from build123d import *

# Parameters (mm, degrees)
SKETCH1_R           = 4
BOSS_EXTRUDE1_DEPTH = 15
CUT_EXTRUDE1_REACH  = 83.718
FILLET1_R           = 5


with BuildPart() as part:
    # Sketch1 → Boss-Extrude1 (new, symmetric)
    with BuildSketch(Plane.XY):
        with BuildLine():
            Line((-32.411165235, -2.9), (32.411165235, -2.9))
            ThreePointArc((32.411165235, -2.9), (36.084926186, -3.630756488), (39.199390335, -5.711774901))
            Line((39.199390335, -5.711774901), (51.448127676, -17.960512242))
            ThreePointArc((51.448127676, -17.960512242), (54.259902577, -24.748737342), (51.448127676, -31.536962441))
            Line((51.448127676, -31.536962441), (44.756401435, -38.228688682))
            ThreePointArc((44.756401435, -38.228688682), (38.472718241, -48.613591207), (48.857620766, -42.329908013))
            Line((48.857620766, -42.329908013), (55.549347007, -35.638181772))
            ThreePointArc((55.549347007, -35.638181772), (60.059902577, -24.748737342), (55.549347007, -13.859292911))
            Line((55.549347007, -13.859292911), (43.300609665, -1.61055557))
            ThreePointArc((43.300609665, -1.61055557), (38.304490094, 1.727744801), (32.411165235, 2.9))
            Line((32.411165235, 2.9), (-32.411165235, 2.9))
            Line((-32.411165235, 2.9), (-32.411165235, -2.9))
        make_face()
        with Locations((42.892135624, -44.194173824)):
            Circle(SKETCH1_R, mode=Mode.SUBTRACT)
    extrude(amount=BOSS_EXTRUDE1_DEPTH, both=True)

    # Sketch2 → Cut-Extrude1 (cut, up to next)
    with BuildSketch(Plane(origin=(0, 2.9, 0), x_dir=(1, 0, 0), z_dir=(0, 1, 0)), mode=Mode.PRIVATE) as cut_extrude1_sk1:
        with BuildLine():
            Line((-2.411165235, 3.5), (6.588834765, 3.5))
            ThreePointArc((6.588834765, 3.5), (10.088834765, 0), (6.588834765, -3.5))
            Line((6.588834765, -3.5), (-2.411165235, -3.5))
            ThreePointArc((-2.411165235, -3.5), (-5.911165235, 0), (-2.411165235, 3.5))
        make_face()
    cut_extrude1_tool1 = extrude(cut_extrude1_sk1.sketch, amount=-CUT_EXTRUDE1_REACH, mode=Mode.PRIVATE) & part.part
    add(cut_extrude1_tool1.solids().sort_by_distance((2.088835, 2.9, 0))[0], mode=Mode.SUBTRACT)

    # Fillet1
    fillet1_edges = [part.edges().sort_by_distance(p)[0] for p in [
        (-32.411165235, 0, -15),
        (-32.411165235, 0, 15),
    ]]
    fillet(fillet1_edges, radius=FILLET1_R)


solid = part.part
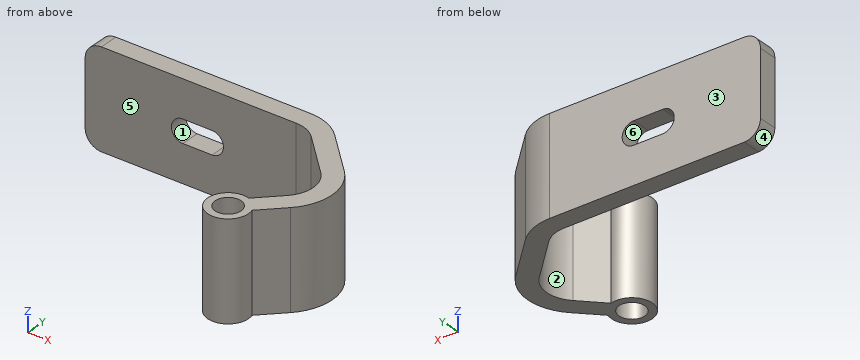
Here's how the part is built. I have some questions about the finished solid (model axes, mm). Face numbers are marked on the shaded views. A direction names the side the tool comes from. Round coordinates to 2 decimals unless told otherwise and drop trailing zeros. Order: outer loops, then holes, each group sorted by start corner. A loop starts at its lowest first (then second) coordinate and runs counter-clockwise, first axis right, second up. Notation, with made-up numbers: M 22,9.5 L 46,9.5 A25 ccw 46,38.5 Z; hole C 28,-24.5 d8. An arc over 180 degrees is marked long. Return JSON: item names as keys, results as strings. Group by question number.
1. I'm going to push flat-ended pins straight in: pin 1 Ø2 at (y, z) = (-7, 9) entering from -X; pin 2 Ø9 at (x, z) = (-8, 0.5) entering from -Y; pin 3 Ø6 at (y, z) = (-29.5, -7) entering from -X; pin 4 Ø7 at (x, y) = (42.89, -44.19) entering from +Z. Where does each tip first touch, or does it pass through?
2. If we mould it in two halves opening along Y, with no side actions, what happens to the marked faces 1, 2 and 3? For each: pulls with the +Y half, pulls with the -Y half, needs draft (parallel to the pull), parting line crosses it, or undercut.
3. If we section it at B-B on x = 2: List the corners of the cut face in (y, z) for me.
4. On a 3-axis mill with a long thin cutter (end or side, diameter ignored), from which of +Z, -Z, +X, -X, +Y, -Y can I reach the whole of each face in a straight line? I mean the marked faces 4, 5 and 6. Say none if no direction works.
5. If we section it at A-A on z = 0: List the corners of the cut face in (x, y) for me, then the cut area to 3 significant figures.
6. Please list where these lines run through material, in increasing order: probe 1 along Y at (x, z) = (-14.5, -11.5); probe 2 along Y at (x, z) = (46.5, 10.25); probe 3 along Y at (x, z) = (52, -10.5).
7. If we section it at C-C on z = 6.5: List the corners of the cut face in (x, y) for me.
8. If we section it at D-D on x = -19: List the corners of the cut face in (y, z) for me, then the cut area to 3 significant figures.
Reply:
{
 "1": {"pin 1": "x = 39.49", "pin 2": "y = -2.9", "pin 3": "x = 50.49", "pin 4": "through"},
 "2": {"face 1": "needs draft", "face 2": "undercut", "face 3": "pulls with the +Y half"},
 "3": {"outline": "M -2.9,-15 L 2.9,-15 L 2.9,-3.5 L -2.9,-3.5 Z; M -2.9,3.5 L 2.9,3.5 L 2.9,15 L -2.9,15 Z"},
 "4": {"face 4": "-Z, -X, +Y, -Y", "face 5": "+Z, -Z, -X, -Y", "face 6": "+Y, -Y"},
 "5": {"outline": "M -32.41,-2.9 L -5.91,-2.9 L -5.91,2.9 L -32.41,2.9 Z; M 10.09,-2.9 L 32.41,-2.9 A9.6 cw 39.2,-5.71 L 51.45,-17.96 A9.6 cw 51.45,-31.54 L 44.76,-38.23 A6.25 ccw long 48.86,-42.33 L 55.55,-35.64 A15.4 ccw 55.55,-13.86 L 43.3,-1.61 A15.4 ccw 32.41,2.9 L 10.09,2.9 Z; hole C 42.89,-44.19 d8", "area": "679 mm^2"},
 "6": {"probe 1": "-2.9 to 2.9", "probe 2": "-49.3 to -45.92, -42.47 to -36.49, -13.01 to -4.81", "probe 3": "-39.19 to -30.94, -18.56 to -10.31"},
 "7": {"outline": "M -32.41,-2.9 L 32.41,-2.9 A9.6 cw 39.2,-5.71 L 51.45,-17.96 A9.6 cw 51.45,-31.54 L 44.76,-38.23 A6.25 ccw long 48.86,-42.33 L 55.55,-35.64 A15.4 ccw 55.55,-13.86 L 43.3,-1.61 A15.4 ccw 32.41,2.9 L -32.41,2.9 Z; hole C 42.89,-44.19 d8"},
 "8": {"outline": "M -2.9,-15 L 2.9,-15 L 2.9,15 L -2.9,15 Z", "area": "174 mm^2"}
}
